from build123d import *

# Parameters (mm, degrees)
CUT_EXTRUDE1_DEPTH = 0.0635


with BuildPart() as part:
    # Sketch1 → Revolve1 (revolve)
    with BuildSketch(Plane(origin=(0, 0, 0), x_dir=(0, 0, -1), z_dir=(1, 0, 0))):
        Polygon((-3.5687, 3.302), (-3.5687, 4.8895), (-2.4003, 4.8895), (-2.4003, 7.9375), (-2.7813, 7.9375), (-2.7813, 9.1186), (-2.3749, 9.525), (2.3749, 9.525), (2.7813, 9.1186), (2.7813, 7.9375), (2.4003, 7.9375), (2.4003, 4.8895), (3.5687, 4.8895), (3.5687, 3.302), (3.4417, 3.175), (-3.4417, 3.175), align=None)
    revolve(axis=Axis((0, 0, 0), (0, 0, -1)))

    # Sketch2 → Cut-Extrude1 (cut)
    with BuildSketch(Plane.XY.offset(2.7813)):
        Polygon((-1.065389716, 8.689257304), (-0.944927977, 8.700960028), (-0.923812192, 8.485731663), (-0.775238474, 8.71762369), (-0.6318801, 8.731743282), (-0.823194203, 8.43116135), (-0.549325012, 8.108064395), (-0.690520926, 8.094199211), (-0.910837432, 8.352931182), (-0.883615878, 8.075245886), (-1.004077616, 8.063543161), align=None)
        with BuildLine():
            Line((-0.489550779, 8.745205417), (-0.362092846, 8.750802372))
            add(Edge.make_bspline(
                [(-0.362092846, 8.750802372), (-0.353783496, 8.751094885), (-0.337719442, 8.751660387), (-0.314512555, 8.751859917), (-0.293097259, 8.751130036), (-0.273426615, 8.750177126), (-0.25557832, 8.748042626), (-0.239408839, 8.745617462), (-0.225080822, 8.742341467), (-0.212298345, 8.738378299), (-0.200823557, 8.733485202), (-0.189914069, 8.728251603), (-0.179779185, 8.721890908), (-0.169997559, 8.715093426), (-0.160982847, 8.707235014), (-0.152469707, 8.698745309), (-0.144499674, 8.68948952), (-0.137163657, 8.679508609), (-0.130573946, 8.668808831), (-0.124668367, 8.657561061), (-0.119619418, 8.645720508), (-0.115250492, 8.633375845), (-0.111835881, 8.620431699), (-0.109185181, 8.606920008), (-0.107217999, 8.592822714), (-0.106684397, 8.583196649), (-0.106413759, 8.578314391)],
                knots=[0, 0, 0, 0, 2.4944e-05, 4.8222e-05, 6.9602e-05, 8.9225e-05, 0.000107275, 0.000123504, 0.000138253, 0.000151328, 0.000163588, 0.000175649, 0.000187582, 0.000199441, 0.000211348, 0.000223401, 0.000235488, 0.000247954, 0.000260521, 0.000273152, 0.00028603, 0.000299104, 0.000312403, 0.000326149, 0.000340397, 0.00035506, 0.00035506, 0.00035506, 0.00035506], degree=3))
            add(Edge.make_bspline(
                [(-0.106413759, 8.578314391), (-0.106301145, 8.57292907), (-0.106079291, 8.562319767), (-0.106956067, 8.546709533), (-0.108985222, 8.531734852), (-0.112150836, 8.517427274), (-0.116516958, 8.503788963), (-0.121841952, 8.490732201), (-0.128357362, 8.47833375), (-0.136015471, 8.466683627), (-0.144501712, 8.455688158), (-0.154040626, 8.445647342), (-0.164159304, 8.436201955), (-0.175157805, 8.427603876), (-0.187090246, 8.420035009), (-0.19964346, 8.412982658), (-0.213097771, 8.406836734), (-0.222481909, 8.403469396), (-0.227257109, 8.401755898)],
                knots=[0, 0, 0, 0, 1.6155e-05, 3.1827e-05, 4.6848e-05, 6.1445e-05, 7.5727e-05, 8.9758e-05, 0.000103699, 0.00011767, 0.000131538, 0.000145307, 0.000159169, 0.000173037, 0.000187115, 0.000201521, 0.000216207, 0.000231422, 0.000231422, 0.000231422, 0.000231422], degree=3))
            add(Edge.make_bspline(
                [(-0.227257109, 8.401755898), (-0.230428994, 8.40083463), (-0.237276115, 8.398845897), (-0.248567522, 8.396319688), (-0.261647847, 8.394081399), (-0.276541992, 8.392071054), (-0.293213358, 8.390303809), (-0.3117114, 8.388833395), (-0.331976204, 8.387396251), (-0.346105902, 8.38671699), (-0.353443006, 8.386364271)],
                knots=[0, 0, 0, 0, 9.907e-06, 2.1387e-05, 3.4687e-05, 4.9708e-05, 6.6467e-05, 8.4975e-05, 0.000105375, 0.000127411, 0.000127411, 0.000127411, 0.000127411], degree=3))
            Line((-0.353443006, 8.386364271), (-0.341740282, 8.118855257))
            Line((-0.341740282, 8.118855257), (-0.461947614, 8.113639912))
            Line((-0.461947614, 8.113639912), (-0.489550779, 8.745205417))
        make_face()
        with BuildLine():
            Line((-0.358531147, 8.503518718), (-0.32037009, 8.505172364))
            add(Edge.make_bspline(
                [(-0.32037009, 8.505172364), (-0.313456644, 8.505592798), (-0.300711051, 8.506367909), (-0.283338162, 8.508066241), (-0.269442305, 8.510743628), (-0.258483675, 8.513806757), (-0.249827521, 8.518175494), (-0.242563252, 8.523364305), (-0.236339925, 8.529632522), (-0.231078239, 8.53675751), (-0.227040183, 8.54486288), (-0.224012592, 8.553649742), (-0.222695566, 8.563264025), (-0.222683841, 8.569831817), (-0.222677782, 8.57322625)],
                knots=[0, 0, 0, 0, 2.0781e-05, 3.8312e-05, 5.2308e-05, 6.3212e-05, 7.2314e-05, 8.1246e-05, 8.9881e-05, 9.8709e-05, 0.000107697, 0.000116949, 0.000126466, 0.000136645, 0.000136645, 0.000136645, 0.000136645], degree=3))
            add(Edge.make_bspline(
                [(-0.222677782, 8.57322625), (-0.222917637, 8.576158471), (-0.22338335, 8.581851802), (-0.224998846, 8.590031341), (-0.227597902, 8.59754684), (-0.23099774, 8.604406251), (-0.235304004, 8.610636746), (-0.240375218, 8.61626779), (-0.246452189, 8.62116902), (-0.251005053, 8.62378647), (-0.253333831, 8.625125289)],
                knots=[0, 0, 0, 0, 8.822e-06, 1.7129e-05, 2.4933e-05, 3.2613e-05, 4.0023e-05, 4.7587e-05, 5.5275e-05, 6.3325e-05, 6.3325e-05, 6.3325e-05, 6.3325e-05], degree=3))
            add(Edge.make_bspline(
                [(-0.253333831, 8.625125289), (-0.255266589, 8.626057529), (-0.259374974, 8.628039155), (-0.266333987, 8.630303419), (-0.274399852, 8.632008988), (-0.283527412, 8.633423979), (-0.293729577, 8.634232301), (-0.304971839, 8.634778726), (-0.31732103, 8.634719634), (-0.325925391, 8.634433422), (-0.330419168, 8.634283942)],
                knots=[0, 0, 0, 0, 6.432e-06, 1.3673e-05, 2.1882e-05, 3.1147e-05, 4.1362e-05, 5.2568e-05, 6.4906e-05, 7.8395e-05, 7.8395e-05, 7.8395e-05, 7.8395e-05], degree=3))
            Line((-0.330419168, 8.634283942), (-0.364255306, 8.6327575))
            Line((-0.364255306, 8.6327575), (-0.358531147, 8.503518718))
        make_face(mode=Mode.SUBTRACT)
        Polygon((0.274619381, 8.766223521), (0.394826713, 8.762407416), (0.381979157, 8.355737744), (0.438203115, 8.353956895), (0.434641417, 8.242781013), (0.378417458, 8.244561863), (0.374346945, 8.11494147), (0.256810888, 8.118630372), (0.260881401, 8.248250765), (-0.01476864, 8.257027808), (-0.011206941, 8.36820369), align=None)
        Polygon((0.264443099, 8.359426646), (0.271057683, 8.571093313), (0.120194301, 8.364005973), align=None, mode=Mode.SUBTRACT)
        Polygon((0.774863847, 8.722125534), (0.896852028, 8.710550013), (1.080152309, 8.056087873), (0.955238446, 8.067790598), (0.91822222, 8.202626335), (0.660635081, 8.226922208), (0.596778911, 8.101753939), (0.471737845, 8.113456663), align=None)
        Polygon((0.820911523, 8.548747128), (0.716350225, 8.339878939), (0.884131675, 8.323978498), align=None, mode=Mode.SUBTRACT)
    extrude(amount=-CUT_EXTRUDE1_DEPTH, mode=Mode.SUBTRACT)


solid = part.part
Geometry check sheet. Reference: the model listing, model coordinates, mm. A direction names the side the tool comes from. Give positions to 0.01 mm unless a question says otherwise; leave off trailing zeros. Order: outer loops, then holes, each group sorted by start corner. A loop starts at its lowest first (then second) coordinate and runs counter-clockwise, first axis right, second up. Notation, with made-up numbers: (-18, -23) - (31, -23) arc R28 ccw to (31, 10) - close; hole circle Ø11 at (63.5, 38). An arc over 180 degrees is marked (long way). Answer as a JSON object with one key per item and string values.
(1) Tool access check on faces 1 (the cylindrical face through (-4.773, -1.06, 2.976)), 2 (the cylindrical face through (-3.1, -0.69, 0.05)), 3 (the flat face through (0.1, 5.2, -2.4)). Record the directions out of +Z, -Z, +X, -X, +Y, -Y that give a thin tool (end or side, any length) a straight path to the whole face; none if there is none.
Report:
{"face 1": "+Z", "face 2": "+Z, -Z", "face 3": "-Z"}
(2) Draft check along Y on faces 4 (the cylindrical face through (-5.796, -7.559, -0.033)), 5 (the flat face through (0, -8.1, 2.781)), 6 (the flat face through (0.1, -5.2, 2.4)), 7 (the cylindrical face through (-4.773, -1.06, -2.993)). Enter one of: released by +Y, released by -Y, zero draft, split by the parting line, or undercut.
Report:
{"face 4": "split by the parting line", "face 5": "zero draft", "face 6": "undercut", "face 7": "undercut"}
(3) Material ranges on line 1 (Y direction, x = -0.5, z = -2.75); line 2 (X direction, y = 0, z = -2.5) (1 decimal); line 3 (X direction, y = 0, z = 2.6) (1 decimal), recorded low to high.
Report:
{"line 1": "-9.14 to -7.92, -4.86 to -3.14, 3.14 to 4.86, 7.92 to 9.14", "line 2": "-9.4 to -7.9, -4.9 to -3.2, 3.2 to 4.9, 7.9 to 9.4", "line 3": "-9.3 to -7.9, -4.9 to -3.2, 3.2 to 4.9, 7.9 to 9.3"}
(4) Depth check by flat-ended pin: pin 1 Ø0.5 at (x, y) = (1, 8.5) entering from +Z; pin 2 Ø1.5 at (y, z) = (1, 3) entering from -X; pin 3 Ø1.5 at (y, z) = (7, -1) entering from +X. Enter the tip coordinate at first touch or a pass-through.
Report:
{"pin 1": "z = 2.78", "pin 2": "x = -9.51", "pin 3": "x = 7.19"}
(5) Cross-section at B-B (z = -2). Record the cut outline in (x, y) (3 decimals).
Report:
{"outline": "circle Ø19.05 at (0, 0); hole circle Ø6.35 at (0, 0)"}
